Can you work these out from the model? Positions are in its coordinate system, mm. Give positions to 0.01 mm unless a question says otherwise; leave off trailing zeros. Write each loop counter-clockwise with the first axis right and the second up, starting at its lowest first coordinate (ties: lowest second). Pieces come first, ordered by that corner, then holes.
1. Suppose I cut it at A-A (z = -8). Please give me the cut outline in (x, y), and give its area (3 significant figures).
2. Suppose I cut it at B-B (x = 66). Please give me the cut outline in (y, z).
3. If I drill on probe 1 along Z at (x, y) = (80, 1.9); probe 2 along X at (y, z) = (1.5, -8); probe 3 along X at (y, z) = (3.9, -20), over which ranges is the centre line in solid material (lowest first)?
```python
from build123d import *

# Parameters (mm, degrees)
SKETCH_1_R      = 1.7
EXTRUDE_1_DEPTH = 5


with BuildPart() as part:
    # 草图1 → 凸台-拉伸1 (new body)
    with BuildSketch(Plane(origin=(0, 0, 0), x_dir=(1, 0, 0), z_dir=(0, 1, 0))):
        with BuildLine():
            Line((-85, 25), (85, 25))
            ThreePointArc((85, 25), (88.535533906, 23.535533906), (90, 20))
            Line((90, 20), (90, -20))
            ThreePointArc((90, -20), (88.535533906, -23.535533906), (85, -25))
            Line((85, -25), (-85, -25))
            ThreePointArc((-85, -25), (-88.535533906, -23.535533906), (-90, -20))
            Line((-90, -20), (-90, 20))
            ThreePointArc((-90, 20), (-88.535533906, 23.535533906), (-85, 25))
        make_face()
        with Locations(Location((-85, 20, 0), (0, 0, 270))):
            Circle(SKETCH_1_R, mode=Mode.SUBTRACT)
        with Locations(Location((-85, -20, 0), (0, 0, 270))):
            Circle(SKETCH_1_R, mode=Mode.SUBTRACT)
        with Locations(Location((85, 20, 0), (0, 0, 270))):
            Circle(SKETCH_1_R, mode=Mode.SUBTRACT)
        with Locations(Location((85, -20, 0), (0, 0, 270))):
            Circle(SKETCH_1_R, mode=Mode.SUBTRACT)
        with Locations(Location((-80, 8, 0), (0, 0, 270))):
            Circle(SKETCH_1_R, mode=Mode.SUBTRACT)
        with Locations(Location((-80, -8, 0), (0, 0, 270))):
            Circle(SKETCH_1_R, mode=Mode.SUBTRACT)
        with Locations(Location((-66, -8, 0), (0, 0, 90))):
            Circle(SKETCH_1_R, mode=Mode.SUBTRACT)
        with Locations(Location((-66, 8, 0), (0, 0, 90))):
            Circle(SKETCH_1_R, mode=Mode.SUBTRACT)
        with Locations(Location((66, -8, 0), (0, 0, 270))):
            Circle(SKETCH_1_R, mode=Mode.SUBTRACT)
        with Locations(Location((66, 8, 0), (0, 0, 270))):
            Circle(SKETCH_1_R, mode=Mode.SUBTRACT)
        with Locations(Location((80, -8, 0), (0, 0, 90))):
            Circle(SKETCH_1_R, mode=Mode.SUBTRACT)
        with Locations(Location((80, 8, 0), (0, 0, 90))):
            Circle(SKETCH_1_R, mode=Mode.SUBTRACT)
    extrude(amount=EXTRUDE_1_DEPTH)


solid = part.part
```
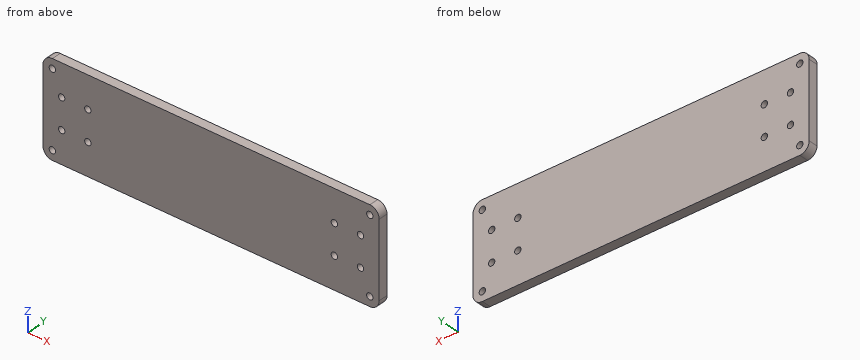
Checks:
1. outline: (-90, 0) - (-81.7, 0) - (-81.7, 5) - (-90, 5) - close; (-78.3, 0) - (-67.7, 0) - (-67.7, 5) - (-78.3, 5) - close; (-64.3, 0) - (64.3, 0) - (64.3, 5) - (-64.3, 5) - close; (67.7, 0) - (78.3, 0) - (78.3, 5) - (67.7, 5) - close; (81.7, 0) - (90, 0) - (90, 5) - (81.7, 5) - close
1. area: 832 mm2
2. outline: (0, -25) - (5, -25) - (5, -9.7) - (0, -9.7) - close; (0, -6.3) - (5, -6.3) - (5, 6.3) - (0, 6.3) - close; (0, 9.7) - (5, 9.7) - (5, 25) - (0, 25) - close
3. probe 1: z = -25 to -9.7, -6.3 to 6.3, 9.7 to 25
3. probe 2: x = -90 to -81.7, -78.3 to -67.7, -64.3 to 64.3, 67.7 to 78.3, 81.7 to 90
3. probe 3: x = -90 to -86.7, -83.3 to 83.3, 86.7 to 90
